Here's how the part is built. I have some questions about the finished solid (model axes, mm). Face numbers are marked on the shaded views. Round coordinates to 2 decimals unless told otherwise and drop trailing zeros. Loops run counter-clockwise (first coordinate to the right, second up) from the corner with the lowest first, then second, coordinate; pieces in that order, holes last. Notation, with made-up numbers: M -22.75,65 L 29.25,65 A14 ccw 29.25,72 Z; hole C -22,-28 d10. An arc over 180 degrees is marked long. Answer as a JSON object with one key per item and string values.
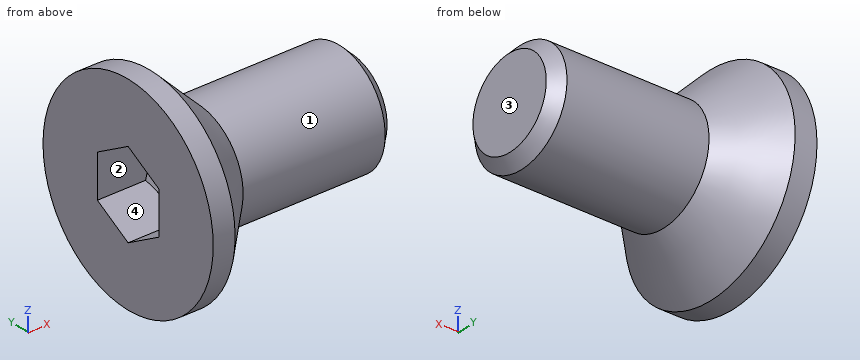
Autodesk Inventor part; units mm, degrees
ref_plane "Work Plane1" through (104.775, 0, 0) normal (0, 0, -1) x (1, 0, 0)
ref_plane "YZ Plane" through (0, 0, 0) normal (1, 0, 0) x (0, 1, 0)
ref_plane "XZ Plane" through (0, 0, 0) normal (0, 1, 0) x (-1, 0, 0)
sketch "Skizze1" plane through (0, 0, 0) normal (0, 0, 1) x (1, 0, 0)
  line L0 (6, 0) -> (6, 1.5)
  line L1 (6, 1.5) -> (2.5, 1.5)
  line L2 (2.5, 1.5) -> (2.1933, 1.5)
  line L3 (0, 2.77) -> (0, 1.1547)
  line L4 (0, 1.1547) -> (1.3, 1.1547)
  line L5 (1.3, 1.1547) -> (1.9667, 0)
  line L6 (1.9667, 0) -> (6, 0)
  line L7 (0, 2.77) -> (0.59, 2.77)
  line L8 (0.59, 2.77) -> (1.86, 1.5)
  line L9 (2.1933, 1.5) -> (1.86, 1.5)
  line L10 (2.5, 1.5) -> (1.86, 1.5) construction
  line L11 (1.86, 1.5) -> (1.86, 1.5)
  line L12 (-1.2, 0) -> (7.2, 0)
  line L13 (0, -0.554) -> (0, 3.324)
  dimension "d0" = 6
  dimension "d1" = 3.5
  dimension "d2" = 1.3
  dimension "d3" = 3
  dimension "d6" = 1.86
  dimension "d7" = 45
  dimension "d8" = 2.3094
  dimension "d9" = 60
  dimension "d10" = 5.54
  dimension "d11" = 3
  dimension "d12" = 0.3067
revolve "Körper" add sketch "Skizze1" angle 360 about axis through (1.9667, 0, 0) along (1, 0, 0) contours L6 L5 L4 L3 L7 L8 L9 L2 L1 L0
sketch "Skizze2" plane through (0, 0, 0) normal (-1, 0, 0) x (0, 0, 1)
  circle A0 centre (0, 0) radius 1.1547
  line L0 (0, -3.878) -> (0, 3.878)
  line L1 (-3.878, 0) -> (3.878, 0)
  line L2 (1.1547, 0) -> (0.5774, -1)
  line L3 (0.5774, -1) -> (-0.5774, -1)
  line L4 (-0.5774, -1) -> (-1.1547, 0)
  line L5 (-1.1547, 0) -> (-0.5774, 1)
  line L6 (-0.5774, 1) -> (0.5774, 1)
  line L7 (0.5774, 1) -> (1.1547, 0)
  point P0 (0, 1.1547)
extrude "Loch" add sketch "Skizze2" against normal up to next contours L7 A0 | A0 L2 | L6 L0 A0 | A0 L0 L3 | L0 L6 A0 | A0 L3 L0 | L4 A0 | A0 L5
thread "Gewinde"
chamfer "Fase1" distance 0.3067 distance2 0.3067 1 edges at (6, -1.5, 0) measured on face at (6, -0.3743, -0.4914)
ref_plane "Work Plane1" through (104.775, 0, 0) normal (0, 0, -1) x (1, 0, 0)
equation "\"d15\" = GEL"
equation "\"d17\" = -0.5 * SPD + 0.5 * GD"
equation "\"d18\" = GUL"
equation "\"d2\" = INTI"
equation "\"d3\" = GD"
equation "\"d6\" = KOH"
equation "\"d7\" = 0.5 * SEWI"
equation "\"d8\" = 1.1547 * SW"
equation "\"d10\" = KOD"
equation "\"d11\" = BDM"
equation "\"d12\" = GAL"
equation "\"NLG\" = 8"
equation "\"INTI\" = 1.3"
equation "\"GEL\" = 4"
equation "\"GAL\" = 0.61345 * PTC"
equation "\"KOH\" = 1.86"
equation "\"KOD\" = 5.54"
equation "\"GUL\" = 0.61345 * PTC"
equation "\"SPD\" = NND - 1.2269 * PTC"
equation "\"BDM\" = NND"
equation "\"GD\" = NND"
equation "\"SEWI\" = 90deg"
equation "\"SW\" = 2"
equation "\"TOA\" = 30deg"
equation "\"GD1\" = THREADDIA - 1.2269 * PTC"
equation "\"EPV\" = 3.36"
equation "\"THREADDIA\" = 3"
equation "\"PTC\" = 0.5"
equation "\"NND\" = 3"
equation "\"E0\" = 2.31"
equation "\"THREADDESC\" = 1.2345"
properties part number "ISO 10642 - M3 x  8" material "Stahl"
Item 1: We'd pull the mould along Y, two halves only. Please class the marked faces 1, 2, 3 and 4: +Y half, -Y half, draft (parallel to the pull), parting line (faces both ways), or undercut.
Solution:
{"face 1": "parting line", "face 2": "undercut", "face 3": "draft", "face 4": "undercut"}
Item 2: I want a section at C-C on x = 1.65. List the corners of the cut face in (y, z) for me.
Solution:
{"outline": "C 0,0 d3.42; hole C 0,0 d1.1"}
Item 3: If I drill on L1, parallel to Y at x = 1, z = -0.55; L2, parallel to X at y = -0.25, z = -1.2; L3, parallel to Y at x = 2.45, z = 0.15, over which ranges is the centre line in solid material (lowest first)? Write a range as from..to.
Solution:
{"L1": "y = -2.3..-1, 1..2.3", "L2": "x = 0..5.97", "L3": "y = -1.49..1.49"}
Item 4: I want a section at B-B on x = 5.2. List the corners of the cut face in (y, z) for me, plus the area to 3 significant figures.
Solution:
{"outline": "C 0,0 d3", "area": "7.07 mm2"}
Item 5: I want a section at A-A on x = 0.4. List the corners of the cut face in (y, z) for me.
Solution:
{"outline": "C 0,0 d5.54; hole M -1,-0.58 L 0,-1.15 L 1,-0.58 L 1,0.58 L 0,1.15 L -1,0.58 Z"}
Item 6: For P1, Ø1, axis at y = 1.5, z = -1, coming from the +X side; P2, Ø0.9, axis at x = 1, z = 0, coming from the -Y side; P3, Ø0.6, axis at x = 1, z = 0, coming from the +Y side, each with a flat end and sliding along its axis, tell me the tip position at first contact or that it passes through.
Solution:
{"P1": "stops at x = 5.89", "P2": "stops at y = -2.77", "P3": "stops at y = 2.66"}
